The model under review builds one solid part; all positions refer to its coordinate system, in mm. A direction names the side the tool comes from. Coordinates: 2 decimals unless noted, no trailing zeros. Write each loop counter-clockwise with the first axis right and the second up, starting at its lowest first coordinate (ties: lowest second). Pieces come first, ordered by that corner, then holes. Notation, with made-up numbers: (50.5, -4.75) - (108.5, -4.75) arc R19 cw to (108.5, 19.25) - close; hole circle Ø9 at (-31, 80). An arc over 180 degrees is marked (long way). Put each result on its own line as item: value.
from build123d import *

# Parameters (mm, degrees)
SKETCH_1_R      = 31.5
SKETCH_1_R_2    = 4
EXTRUDE_1_DEPTH = 12.5
FILLET_1_R      = 2
EXTRUDE_2_DEPTH = 10


with BuildPart() as part:
    # 草图1 → 凸台-拉伸1 (new body)
    with BuildSketch(Plane(origin=(0, 0, 0), x_dir=(1, 0, 0), z_dir=(0, 1, 0))):
        with Locations(Location((0, 0, 0), (0, 0, 270))):
            Circle(SKETCH_1_R)
        with Locations(Location((-15.909902577, 15.909902577, 0), (0, 0, 270))):
            Circle(SKETCH_1_R_2, mode=Mode.SUBTRACT)
        with Locations(Location((15.909902577, 15.909902577, 0), (0, 0, 270))):
            Circle(SKETCH_1_R_2, mode=Mode.SUBTRACT)
        with Locations(Location((15.909902577, -15.909902577, 0), (0, 0, 270))):
            Circle(SKETCH_1_R_2, mode=Mode.SUBTRACT)
        with Locations(Location((-15.909902577, -15.909902577, 0), (0, 0, 270))):
            Circle(SKETCH_1_R_2, mode=Mode.SUBTRACT)
    extrude(amount=EXTRUDE_1_DEPTH)

    # 圆角1
    fillet_1_edges = [part.edges().sort_by_distance(p)[0] for p in [
        (0, 12.5, -31.5),
    ]]
    fillet(fillet_1_edges, radius=FILLET_1_R)

    # 草图2 → 凸台-拉伸2 (add)
    with BuildSketch(Plane(origin=(0, 12.5, 0), x_dir=(1, 0, 0), z_dir=(0, 1, 0))):
        with BuildLine():
            Line((3, 31.356817441), (3, 3))
            Line((3, 3), (31.356817441, 3))
            ThreePointArc((31.356817441, 3), (31.5, 0), (31.356817441, -3))
            Line((31.356817441, -3), (3, -3))
            Line((3, -3), (3, -31.356817441))
            ThreePointArc((3, -31.356817441), (0, -31.5), (-3, -31.356817441))
            Line((-3, -31.356817441), (-3, -3))
            Line((-3, -3), (-31.356817441, -3))
            ThreePointArc((-31.356817441, -3), (-31.5, 0), (-31.356817441, 3))
            Line((-31.356817441, 3), (-3, 3))
            Line((-3, 3), (-3, 31.356817441))
            ThreePointArc((-3, 31.356817441), (0, 31.5), (3, 31.356817441))
        make_face()
    extrude(amount=EXTRUDE_2_DEPTH)


solid = part.part
1. Machinability: for faces 4 (the flat face through (-10, 12.5, -13)), 5 (the flat face through (13, 12.5, 10)), 6 (the flat face through (13, 12.5, -11)), which of the approach directions +Z, -Z, +X, -X, +Y, -Y give a long, thin tool a straight path to every point of the face, cutting with its end or side? Answer none if there is none.
Determined:
face 4: -Z, -X, +Y
face 5: +Z, +X, +Y
face 6: -Z, +X, +Y
2. To check wall thickness, follow probe 1 along Z at (x, y) = (-14.5, 11.5); probe 2 along Y at (x, z) = (8.5, -18); probe 3 along Z at (x, y) = (-11.5, 13). State the ranges of each line that lie inside material, in increasing order.
Determined:
probe 1: z = -27.66 to -19.65, -12.17 to 12.17, 19.65 to 27.66
probe 2: y = 0 to 12.5
probe 3: z = -3 to 3
3. Consider section C-C on z = -18. Give the number of separate pieces and of enclosed holes in the cut face, plus the area to 3 significant figures.
Determined:
separate pieces: 3
enclosed holes: 0
area: 534 mm^2
4. Consider section B-B on y = 4.5. State the section outline as (x, z) points, plus the area to 3 significant figures.
Determined:
outline: circle Ø63 at (0, 0); hole circle Ø8 at (-15.91, -15.91); hole circle Ø8 at (-15.91, 15.91); hole circle Ø8 at (15.91, -15.91); hole circle Ø8 at (15.91, 15.91)
area: 2,920 mm^2
5. The part is to be moulded in two halves that separate along X. For faces 1 (the cylindrical face through (-19.815, 6.162, -16.777)), 2 (the flat face through (-3, 17, 17)), 3 (the cylindrical face through (0, 17.4, -31.5)), say which applies: +X half, -X half, draft (parallel to the pull), parting line (faces both ways), or undercut.
Determined:
face 1: undercut
face 2: -X half
face 3: parting line
6. Consider section A-A on y = 17.5. State the section outline as (x, z) points.
Determined:
outline: (-31.36, -3) - (-3, -3) - (-3, -31.36) arc R31.5 ccw to (3, -31.36) - (3, -3) - (31.36, -3) arc R31.5 ccw to (31.36, 3) - (3, 3) - (3, 31.36) arc R31.5 ccw to (-3, 31.36) - (-3, 3) - (-31.36, 3) arc R31.5 ccw to start
7. For pin 1 Ø5 at (y, z) = (15, 0) entering from +X; pin 2 Ø5 at (x, y) = (-20, 18) entering from +Z; pin 3 Ø0.6 at (x, z) = (-31, 0.5) entering from -Y; pin 4 Ø11 at (x, y) = (-15.5, 19.5) entering from -Z, all flat-tipped, find the tip position at first contact; note any pin that passes through.
Determined:
pin 1: stops at x = 31.5
pin 2: stops at z = 3
pin 3: stops at y = 0
pin 4: stops at z = -3
